```python
from build123d import *

# Parameters (mm, degrees)
SKETCH1_W           = 24.699999876
SKETCH1_H           = 29.87499994
SKETCH1_R           = 1.524
BOSS_EXTRUDE1_DEPTH = 21.082
FILLET1_R           = 1.27


with BuildPart() as part:
    # Sketch1 → Boss-Extrude1 (new body)
    with BuildSketch(Plane(origin=(0, 0, 0), x_dir=(1, 0, 0), z_dir=(0, 1, 0))):
        with Locations((12.349999938, 14.93749997)):
            Rectangle(SKETCH1_W, SKETCH1_H)
        with Locations((12.349999938, 15.875)):
            Circle(SKETCH1_R, mode=Mode.SUBTRACT)
        with Locations((12.349999938, 23.875000002)):
            Circle(SKETCH1_R, mode=Mode.SUBTRACT)
    extrude(amount=BOSS_EXTRUDE1_DEPTH)

    # Fillet1
    fillet1_edges = [part.edges().sort_by_distance(p)[0] for p in [
        (0, 10.541, -29.87499994),
        (24.699999876, 10.541, -29.87499994),
        (24.699999876, 10.541, 0),
        (0, 10.541, 0),
    ]]
    fillet(fillet1_edges, radius=FILLET1_R)


solid = part.part
```
Source: CAD feature listing. Evaluate the final solid. Frame: model axes, mm. Give positions to 0.01 mm unless a question says otherwise; leave off trailing zeros. Loops run counter-clockwise (first coordinate to the right, second up) from the corner with the lowest first, then second, coordinate; pieces in that order, holes last. Notation, with made-up numbers: (12, 22) -> (60, 22) arc R27 cw to (60, 58) -> close; hole circle Ø1 at (-37, 10). An arc over 180 degrees is marked (long way). Put each result on its own line as item: value. Start each with the question number.
1) Contact query for a flat-ended pin moving along its axis: P1, Ø2.5, axis at x = 12.35, z = -23.875, coming from the -Y side (3 decimals). Output: stop coordinate, or through.
2) Material intervals for probe 1 along Z at (x, y) = (12.35, 14) (3 decimals); probe 2 along X at (y, z) = (18.25, -15.75); probe 3 along X at (y, z) = (20.25, -24.25), sorted ascending.
3) Draft query along X for faces 1 (the face through (12, 10, 0)), 2 (the face through (13.17, 10.39, -25.16)), 3 (the face through (0.362, 10.689, -0.382)). Return one class per face: released by +X, released by -X, zero draft, split by the parting line, or undercut.
4) Cut plane A-A (x = 12.35). Return loops of the section in (y, z) (3 decimals), then the cut area to 3 significant figures.
5) Cut plane B-B (y = 18). Return loops of the section in (x, z) (3 decimals).
Results are:
1. P1: passes through
2. probe 1: z = -29.875 to -25.399, -22.351 to -17.399, -14.351 to 0
2. probe 2: x = 0 to 10.83, 13.87 to 24.7
2. probe 3: x = 0 to 10.87, 13.83 to 24.7
3. face 1: zero draft
3. face 2: undercut
3. face 3: released by -X
4. outline: (0, -29.875) -> (21.082, -29.875) -> (21.082, -25.399) -> (0, -25.399) -> close; (0, -22.351) -> (21.082, -22.351) -> (21.082, -17.399) -> (0, -17.399) -> close; (0, -14.351) -> (21.082, -14.351) -> (21.082, 0) -> (0, 0) -> close
4. area: 501 mm2
5. outline: (0, -28.605) arc R1.27 ccw to (1.27, -29.875) -> (23.43, -29.875) arc R1.27 ccw to (24.7, -28.605) -> (24.7, -1.27) arc R1.27 ccw to (23.43, 0) -> (1.27, 0) arc R1.27 ccw to (0, -1.27) -> close; hole circle Ø3.048 at (12.35, -23.875); hole circle Ø3.048 at (12.35, -15.875)
